Can you work these out from the drawing? Everything is in mm from the part's minimum corner. A direction names the side the tool comes from. Round coordinates to 2 decimals unless told otherwise and drop trailing zeros. Loops run counter-clockwise (first coordinate to the right, second up) from the corner with the lowest first, then second, coordinate; pieces in that order, holes last. Notation, with made-up numbers: M 88.25,-37 L 112.25,-37 A19 cw 112.25,-18 Z; hole C -34,68 d9. An arc over 180 degrees is marked long. Use a Markdown table: item, result.
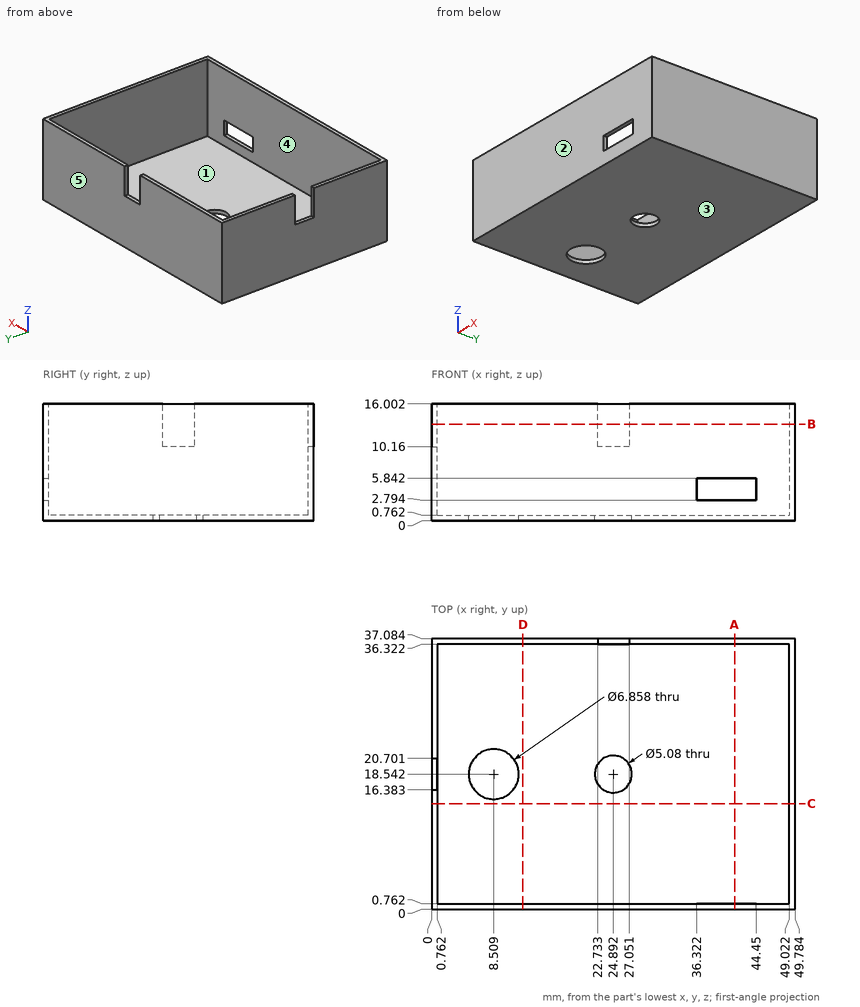
Q1. For the marked faces 4 and 5, which set-ups out of +Z, -Z, +X, -X, +Y, -Y let a thin tool reach every point of the face, with its end or its side?
Return value:
| item | result |
|---|---|
| face 4 | +Z |
| face 5 | +Z, -Z, +X, -X, +Y |
Q2. Imagine slicing it at C-C, the plane y = 14.5. Please give me the cut outline in (x, z).
Return value:
| item | result |
|---|---|
| outline | M 0,0 L 49.78,0 L 49.78,16 L 49.02,16 L 49.02,0.76 L 0.76,0.76 L 0.76,16 L 0,16 Z |
Q3. We'd pull the mould along Y, two halves only. Please class the marked faces 1, 2 and 3: pulls with the +Y half, pulls with the -Y half, needs draft (parallel to the pull), parting line crosses it, or undercut.
Return value:
| item | result |
|---|---|
| face 1 | undercut |
| face 2 | pulls with the -Y half |
| face 3 | needs draft |
Q4. I need wall thicknesses on line 1 (X direction, y = 23.5, z = 9); line 2 (Y direction, x = 7, z = 7); line 3 (Z direction, x = 38, y = 17). Which ranges of each line are inside material? Lowest first, please. Write a range as from..to.
Return value:
| item | result |
|---|---|
| line 1 | x = 0..0.76, 49.02..49.78 |
| line 2 | y = 0..0.76, 36.32..37.08 |
| line 3 | z = 0..0.76 |
Q5. Will these pins go through, and if not, where does the flat tip stop? P1, Ø0.6, axis at x = 24, y = 36.5, coming from the +Z side; P2, Ø6, axis at x = 44.5, y = 14, coming from the +Z side; P3, Ø6, axis at x = 8.509, y = 18.542, coming from the +Z side.
Return value:
| item | result |
|---|---|
| P1 | stops at z = 10.16 |
| P2 | stops at z = 0.76 |
| P3 | passes through |
Q6. Imagine slicing it at D-D, the plane x = 12.5. Please give me the cut outline in (y, z).
Return value:
| item | result |
|---|---|
| outline | M 0,0 L 37.08,0 L 37.08,16 L 36.32,16 L 36.32,0.76 L 0.76,0.76 L 0.76,16 L 0,16 Z |
Q7. Imagine slicing it at B-B, the plane z = 13.25. Please give me the cut outline in (x, y), then the cut area to 3 significant figures.
Return value:
| item | result |
|---|---|
| outline | M 0,0 L 49.78,0 L 49.78,37.08 L 27.05,37.08 L 27.05,36.32 L 49.02,36.32 L 49.02,0.76 L 0.76,0.76 L 0.76,16.38 L 0,16.38 Z; M 0,20.7 L 0.76,20.7 L 0.76,36.32 L 22.73,36.32 L 22.73,37.08 L 0,37.08 Z |
| area | 123 mm^2 |
Q8. Imagine slicing it at A-A, the plane x = 41.5. Please give me the cut outline in (y, z), then the cut area to 3 significant figures.
Return value:
| item | result |
|---|---|
| outline | M 0,0 L 37.08,0 L 37.08,16 L 36.32,16 L 36.32,0.76 L 0.76,0.76 L 0.76,2.79 L 0,2.79 Z; M 0,5.84 L 0.76,5.84 L 0.76,16 L 0,16 Z |
| area | 49.2 mm^2 |
